from build123d import *

# Parameters (mm, degrees)
F0_W     = 75
F0_H     = 20
F1_DEPTH = 24
F2_W     = 71
F2_H     = 20
F3_DEPTH = 20
F5_W     = 5
F5_H     = 11
F6_DEPTH = 5
F7_R     = 1


with BuildPart() as f1:
    # F0 (on Front) → F1 (new body)
    with BuildSketch(Plane.XZ):
        with Locations((37.5, -10)):
            Rectangle(F0_W, F0_H)
    extrude(amount=F1_DEPTH)

    # F2 (on Top) → F3 (cut, symmetric)
    with BuildSketch(Plane.XY):
        with Locations((37.5, -12)):
            Rectangle(F2_W, F2_H)
    extrude(amount=F3_DEPTH, both=True, mode=Mode.SUBTRACT)

    # F5 (on offset) → F6 (cut)
    with BuildSketch(Plane(origin=(0, -22, 0), x_dir=(-1, 0, 0), z_dir=(0, 1, 0))):
        with Locations((-25, -10)):
            Rectangle(F5_W, F5_H)
        with Locations((-50, -9.9999997467)):
            Rectangle(F5_W, F5_H)
    extrude(amount=-F6_DEPTH, mode=Mode.SUBTRACT)

    # F7
    f7_edges = [f1.edges().sort_by_distance(p)[0] for p in [
        (75, -12, -20),
        (75, -12, 0),
        (75, 0, -10),
        (75, -24, -10),
        (37.5, 0, 0),
        (0, 0, -10),
        (37.5, 0, -20),
        (0, -12, 0),
        (0, -12, -20),
        (0, -24, -10),
    ]]
    fillet(f7_edges, radius=F7_R)


solid = f1.part
Could you check a few things on this model? Use its own coordinates, in mm. A direction names the side the tool comes from. Give positions to 0.01 mm unless a question says otherwise; leave off trailing zeros. Write each loop counter-clockwise with the first axis right and the second up, starting at its lowest first coordinate (ties: lowest second). Pieces come first, ordered by that corner, then holes. Notation, with made-up numbers: (17.25, 23.25) -> (27.25, 23.25) arc R7 cw to (27.25, 34.25) -> close; hole circle Ø9 at (28.25, -12.75). An arc over 180 degrees is marked (long way). Answer as a JSON object with one key per item and string values.
Q1. Suppose I cut it at D-D on x = 6. Write out the boundary of the cut face in (y, z).
Taken from the geometry:
{"outline": "(-24, -20) -> (-22, -20) -> (-22, 0) -> (-24, 0) -> close; (-2, -20) -> (-1, -20) arc R1 ccw to (0, -19) -> (0, -1) arc R1 ccw to (-1, 0) -> (-2, 0) -> close"}
Q2. Please list where these lines run through material, in increasing order: L1, parallel to Y at x = 40, z = -2.5; L2, parallel to X at y = -5, z = -5.5.
Taken from the geometry:
{"L1": "y = -24 to -22, -2 to 0", "L2": "x = 0 to 2, 73 to 75"}
Q3. Which directions (+Z, -Z, +X, -X, +Y, -Y) give clear straight access to the entire face, cutting with the end or side of a thin tool? Please do faces 5 (the flat face through (37, -22, -10)), 6 (the flat face through (25, -23, -15.5)), 7 (the flat face through (37, -23, 0)).
Taken from the geometry:
{"face 5": "+Z, -Z", "face 6": "-Y", "face 7": "+Z, +X, -X, +Y, -Y"}
Q4. We'd pull the mould along X, two halves only. Please class faces 1 (the flat face through (2, -12, -10)), 2 (the flat face through (37, -23, -20)), 3 (the flat face through (25, -23, -4.5)), 4 (the flat face through (0, -12, -10)): released by +X, released by -X, zero draft, split by the parting line, or undercut.
Taken from the geometry:
{"face 1": "undercut", "face 2": "zero draft", "face 3": "undercut", "face 4": "released by -X"}
Q5. Suppose I cut it at B-B on y = -7. Write out the boundary of the cut face in (x, z).
Taken from the geometry:
{"outline": "(0, -19) arc R1 ccw to (1, -20) -> (2, -20) -> (2, 0) -> (1, 0) arc R1 ccw to (0, -1) -> close; (73, -20) -> (74, -20) arc R1 ccw to (75, -19) -> (75, -1) arc R1 ccw to (74, 0) -> (73, 0) -> close"}
Q6. Suppose I cut it at A-A on x = 51. Write out the boundary of the cut face in (y, z), then the cut area to 3 significant figures.
Taken from the geometry:
{"outline": "(-24, -20) -> (-22, -20) -> (-22, -15.5) -> (-24, -15.5) -> close; (-24, -4.5) -> (-22, -4.5) -> (-22, 0) -> (-24, 0) -> close; (-2, -20) -> (-1, -20) arc R1 ccw to (0, -19) -> (0, -1) arc R1 ccw to (-1, 0) -> (-2, 0) -> close", "area": "57.6 mm²"}
Q7. Suppose I cut it at C-C on z = -6.25. Write out the boundary of the cut face in (x, y), then the cut area to 3 significant figures.
Taken from the geometry:
{"outline": "(0, -23) arc R1 ccw to (1, -24) -> (22.5, -24) -> (22.5, -22) -> (2, -22) -> (2, -2) -> (73, -2) -> (73, -22) -> (52.5, -22) -> (52.5, -24) -> (74, -24) arc R1 ccw to (75, -23) -> (75, -1) arc R1 ccw to (74, 0) -> (1, 0) arc R1 ccw to (0, -1) -> close; (27.5, -24) -> (47.5, -24) -> (47.5, -22) -> (27.5, -22) -> close", "area": "359 mm²"}
